Part model, mm, in its own coordinate system. Round coordinates to 2 decimals unless told otherwise and drop trailing zeros. Loops run counter-clockwise (first coordinate to the right, second up) from the corner with the lowest first, then second, coordinate; pieces in that order, holes last.
(1) Flat gauge pins, fed straight in: pin 1 (10.5 mm diameter, centred on x = -0.32, y = 40.94, fed in from -Z); pin 2 (1 mm diameter, centred on y = 8.5, z = -0.5, fed in from -X); pin 3 (1 mm diameter, centred on y = -13.5, z = -2, fed in from +X). Where does each tip first touch, or does it go through?
(2) Cut at B-B on y = 31. List the corners of the cut face in (x, z), then the cut area to 3 significant figures.
(3) Cut at A-A on x = 38.5. List the corners of the cut face in (y, z), then the cut area to 3 significant figures.
(4) Probe probe 1 along Y at (x, z) = (-35.5, -0.2); probe 2 along Y at (x, z) = (34.5, -1.1); probe 3 along X at (y, z) = (24.5, -0.5). List the from-to ranges inside material, lowest first.
(5) Mould opens along Y. For faces 1 (the face through (-1, 0, -2.54)), 2 (the face through (0.836, -47.314, -1.288)) say: +Y half, -Y half, draft (parallel to the pull), parting line (faces both ways), or undercut.
(6) Cut at C-C on z = -1.4. Count the separate pieces of the cut face and the enclosed holes in it, then the cut area to 3 significant figures.
(7) Cut at D-D on x = 17. List the corners of the cut face in (y, z).
from build123d import *

# Parameters (mm, degrees)
F1_DEPTH = 2.54
F2_D     = 11.43
F3_D     = 6.35


with BuildPart() as f1:
    # F0 (on Top) → F1 (new body)
    with BuildSketch(Plane.XY):
        with BuildLine():
            ThreePointArc((14.1469296791, 24.581208667), (28.3570527779, 32.9867129725), (42.7414945684, 24.8831374968))
            ThreePointArc((42.7414945684, 24.8831374968), (24.4218518628, 42.8199500657), (-0.4118303798, 49.1938641112))
            ThreePointArc((-0.4118303798, 49.1938641112), (11.3750266033, 44.4205864041), (16.2724880694, 32.6847843949))
            ThreePointArc((16.2724880694, 32.6847843949), (15.7322599992, 28.495931985), (14.1469296791, 24.581208667))
        make_face()
        with BuildLine():
            ThreePointArc((-14.4476350188, 24.2792801377), (-14.6219536378, 40.7883599496), (-0.4118303798, 49.1938641112))
            ThreePointArc((-0.4118303798, 49.1938641112), (-25.1053870129, 42.2969945819), (-43.0421996808, 23.9773521233))
            ThreePointArc((-43.0421996808, 23.9773521233), (-28.8320764588, 32.3828558193), (-14.4476350188, 24.2792801377))
        make_face()
        with BuildLine():
            ThreePointArc((-28.4834395144, -0.6353036127), (-42.8678814784, 7.4682721021), (-43.0421996808, 23.9773521233))
            ThreePointArc((-43.0421996808, 23.9773521233), (-49.4161139914, -0.8563299278), (-42.5192447927, -25.5498866402))
            ThreePointArc((-42.5192447927, -25.5498866402), (-42.6935625622, -9.0408072614), (-28.4834395144, -0.6353036127))
        make_face()
        with BuildLine():
            ThreePointArc((-42.5192447927, -25.5498866402), (-24.1996024135, -43.4866996437), (0.6340797732, -49.8606141921))
            ThreePointArc((0.6340797732, -49.8606141921), (-13.7503612776, -41.757037972), (-13.9246792181, -25.2479584958))
            ThreePointArc((-13.9246792181, -25.2479584958), (-28.1348028533, -33.6534630478), (-42.5192447927, -25.5498866402))
        make_face()
        with BuildLine():
            ThreePointArc((0.6340797732, -49.8606141921), (25.3276368535, -42.9637449392), (43.2644499105, -24.6441023627))
            ThreePointArc((43.2644499105, -24.6441023627), (29.0543267516, -33.0496058908), (14.6698854093, -24.9460303205))
            ThreePointArc((14.6698854093, -24.9460303205), (16.3844166198, -28.9943010133), (16.969762255, -33.351534466))
            ThreePointArc((16.969762255, -33.351534466), (12.1955639367, -44.9640733309), (0.6340797732, -49.8606141921))
        make_face()
        with BuildLine():
            ThreePointArc((43.2644499105, -24.6441023627), (48.0204409306, -12.8999323449), (49.6411251622, -0.3333750356))
            ThreePointArc((49.6411251622, -0.3333750356), (47.8850882419, 12.7383253763), (42.7414945684, 24.8831374968))
            ThreePointArc((42.7414945684, 24.8831374968), (44.4560258195, 20.8348667633), (45.0413714688, 16.4776332587))
            ThreePointArc((45.0413714688, 16.4776332587), (40.2671733446, 4.86509459), (28.7056895388, -0.0314464615))
            ThreePointArc((28.7056895388, -0.0314464615), (40.4925468917, -4.8047239608), (45.3900085616, -16.5405261717))
            ThreePointArc((45.3900085616, -16.5405261717), (44.8497804239, -20.7293788387), (43.2644499105, -24.6441023627))
        make_face()
        with BuildLine():
            ThreePointArc((14.6698854093, -24.9460303205), (29.0543267516, -33.0496058908), (43.2644499105, -24.6441023627))
            ThreePointArc((43.2644499105, -24.6441023627), (44.8497804239, -20.7293788387), (45.3900085616, -16.5405261717))
            ThreePointArc((45.3900085616, -16.5405261717), (40.4925468917, -4.8047239608), (28.7056895388, -0.0314464615))
            ThreePointArc((28.7056895388, -0.0314464615), (14.4955667445, -8.436950812), (14.6698854093, -24.9460303205))
        make_face()
        with BuildLine():
            ThreePointArc((-13.9246792181, -25.2479584958), (-13.7503612776, -41.757037972), (0.6340797732, -49.8606141921))
            ThreePointArc((0.6340797732, -49.8606141921), (12.1955639367, -44.9640733309), (16.969762255, -33.351534466))
            ThreePointArc((16.969762255, -33.351534466), (16.3844166198, -28.9943010133), (14.6698854093, -24.9460303205))
            ThreePointArc((14.6698854093, -24.9460303205), (0.2854439404, -16.8424547484), (-13.9246792181, -25.2479584958))
        make_face()
        with BuildLine():
            ThreePointArc((-28.4834395144, -0.6353036127), (-42.6935625622, -9.0408072614), (-42.5192447927, -25.5498866402))
            ThreePointArc((-42.5192447927, -25.5498866402), (-28.1348028533, -33.6534630478), (-13.9246792181, -25.2479584958))
            ThreePointArc((-13.9246792181, -25.2479584958), (-12.3393491328, -21.3332354278), (-11.7991211444, -17.1443833299))
            ThreePointArc((-11.7991211444, -17.1443833299), (-16.6965825823, -5.4085813485), (-28.4834395144, -0.6353036127))
        make_face()
        with BuildLine():
            ThreePointArc((-14.4476350188, 24.2792801377), (-28.8320764588, 32.3828558193), (-43.0421996808, 23.9773521233))
            ThreePointArc((-43.0421996808, 23.9773521233), (-42.8678814784, 7.4682721021), (-28.4834395144, -0.6353036127))
            ThreePointArc((-28.4834395144, -0.6353036127), (-16.9219561318, 4.2612376639), (-12.1477582372, 15.8737761006))
            ThreePointArc((-12.1477582372, 15.8737761006), (-12.7331038558, 20.2310094926), (-14.4476350188, 24.2792801377))
        make_face()
        with BuildLine():
            ThreePointArc((16.2724880694, 32.6847843949), (11.3750266033, 44.4205864041), (-0.4118303798, 49.1938641112))
            ThreePointArc((-0.4118303798, 49.1938641112), (-14.6219536378, 40.7883599496), (-14.4476350188, 24.2792801377))
            ThreePointArc((-14.4476350188, 24.2792801377), (-0.0631934119, 16.1757046794), (14.1469296791, 24.581208667))
            ThreePointArc((14.1469296791, 24.581208667), (15.7322599992, 28.495931985), (16.2724880694, 32.6847843949))
        make_face()
        with BuildLine():
            ThreePointArc((45.0413714688, 16.4776332587), (44.4560258195, 20.8348667633), (42.7414945684, 24.8831374968))
            ThreePointArc((42.7414945684, 24.8831374968), (28.3570527779, 32.9867129725), (14.1469296791, 24.581208667))
            ThreePointArc((14.1469296791, 24.581208667), (14.3212482409, 8.0721292377), (28.7056895388, -0.0314464615))
            ThreePointArc((28.7056895388, -0.0314464615), (40.2671733446, 4.86509459), (45.0413714688, 16.4776332587))
        make_face()
        with BuildLine():
            ThreePointArc((28.7056895388, -0.0314464615), (14.3212482409, 8.0721292377), (14.1469296791, 24.581208667))
            ThreePointArc((14.1469296791, 24.581208667), (-0.0631934119, 16.1757046794), (-14.4476350188, 24.2792801377))
            ThreePointArc((-14.4476350188, 24.2792801377), (-12.7331038558, 20.2310094926), (-12.1477582372, 15.8737761006))
            ThreePointArc((-12.1477582372, 15.8737761006), (-16.9219561318, 4.2612376639), (-28.4834395144, -0.6353036127))
            ThreePointArc((-28.4834395144, -0.6353036127), (-16.6965825823, -5.4085813485), (-11.7991211444, -17.1443833299))
            ThreePointArc((-11.7991211444, -17.1443833299), (-12.3393491328, -21.3332354278), (-13.9246792181, -25.2479584958))
            ThreePointArc((-13.9246792181, -25.2479584958), (0.2854439404, -16.8424547484), (14.6698854093, -24.9460303205))
            ThreePointArc((14.6698854093, -24.9460303205), (14.4955667445, -8.436950812), (28.7056895388, -0.0314464615))
        make_face()
    extrude(amount=-F1_DEPTH)

    # F2 (through all)
    with Locations(Plane.XY):
        with Locations((-0.3246712038, 40.9393242526), (35.6364330455, 20.6803853323), (36.0722294115, -20.5923139558), (0.5469215282, -41.6060743237), (-35.4141827211, -21.3471354034), (-35.849979087, 19.9255638847)):
            Hole(F2_D / 2)

    # F3 (through all)
    with Locations(Plane.XY):
        with Locations((-28.6577582372, 15.8737761006), (-0.2375119306, 32.6847843949), (28.5313714688, 16.4776332587), (28.8800085616, -16.5405261717), (0.459762255, -33.351534466), (-28.3091211444, -17.1443833299)):
            Hole(F3_D / 2)


solid = f1.part
Final values:
1. pin 1: passes through
1. pin 2: stops at x = -48.71
1. pin 3: stops at x = 47.99
2. outline: (-38.25, -2.54) - (-2.93, -2.54) - (-2.93, 0) - (-38.25, 0) - close; (2.45, -2.54) - (38.47, -2.54) - (38.47, 0) - (2.45, 0) - close
2. area: 181 mm2
3. outline: (-31.63, -2.54) - (-25.77, -2.54) - (-25.77, 0) - (-31.63, 0) - close; (-15.42, -2.54) - (15.73, -2.54) - (15.73, 0) - (-15.42, 0) - close; (25.63, -2.54) - (30.96, -2.54) - (30.96, 0) - (25.63, 0) - close
3. area: 108 mm2
4. probe 1: y = -34.76 to -27.06, -15.63 to 14.22, 25.63 to 34.09
4. probe 2: y = -35.98 to -26.09, -15.1 to 15.08, 26.28 to 35.31
4. probe 3: x = -42.74 to -39.28, -32.42 to 31.39, 39.89 to 42.97
5. face 1: draft
5. face 2: undercut
6. separate pieces: 1
6. enclosed holes: 6
6. area: 6,910 mm2
7. outline: (-46.9, -2.54) - (46.23, -2.54) - (46.23, 0) - (-46.9, 0) - close
